Verification items for the finished model (mm, model axes). A direction names the side the tool comes from. Coordinates: 2 decimals unless noted, no trailing zeros. Loops run counter-clockwise (first coordinate to the right, second up) from the corner with the lowest first, then second, coordinate; pieces in that order, holes last. Notation, with made-up numbers: (35, 6) - (46, 6) arc R20 cw to (46, 33) - close; hole circle Ø5 at (20, -15.75). An arc over 180 degrees is marked (long way). Answer as CSV lines item,"result". Start each with the question number.
1. Set-up check for faces 1 (the flat face through (2, 5.562, 0)), 2 (the cylindrical face through (2.539, -3.023, 17.085)): record each of +Z, -Z, +X, -X, +Y, -Y from which the full face is reachable in a straight line by a thin tool's end or side.
2. Cross-section at C-C (x = 3.75). State how many separate pieces and enclosed holes the cut face has, plus the area to 3 significant figures.
3. Gauge pin test, flat ends, axial feed: P1, Ø0.8, axis at x = 3.5, z = 0, coming from the -Y side; P2, Ø12, axis at y = -11.5, z = 14, coming from the +X side; P3, Ø1.5, axis at x = 3, y = -6, coming from the +Z side; P4, Ø1.5, axis at y = 0, z = 7.5, coming from the -X side. Record the tip position at first contact, or that the pin passes through.
4. Material ranges on line 1 (Y direction, x = 2.5, z = 0) (3 decimals); line 2 (Z direction, x = 0.35, y = 2.5); line 3 (Z direction, x = 1.85, y = 9), recorded low to high. Write a range as [from, to].
5. Cross-section at A-A (y = 0). Enter the section's corners in (x, z) (3 decimals), plus the area to 3 significant figures.
6. Release check for a two-part mould opening along Y. For faces 3 (the cylindrical face through (2.539, 8.684, -15.02)), 4 (the flat face through (2.46, 2.79, 4.81)), 5 (the flat face through (2.465, 8.988, 3.874)), 6 (the cylindrical face through (2.54, -4.48, -16.76)) record: pulls with the +Y half, pulls with the -Y half, needs draft (parallel to the pull), parting line crosses it, or undercut.
```python
from build123d import *

# Parameters (mm, degrees)
SKETCH1_R           = 20
SKETCH1_R_2         = 1.705
BOSS_EXTRUDE1_DEPTH = 5
CUT_EXTRUDE1_DEPTH  = 8
CIRPATTERN1_COUNT   = 12
CUT_EXTRUDE2_DEPTH  = 2.5
CIRPATTERN2_COUNT   = 71
CIRPATTERN2_ANGLE   = 350


with BuildPart() as part:
    # Sketch1 → Boss-Extrude1 (new body)
    with BuildSketch(Plane(origin=(0, 0, 0), x_dir=(0, 0, -1), z_dir=(1, 0, 0))):
        Circle(SKETCH1_R)
        Circle(SKETCH1_R_2, mode=Mode.SUBTRACT)
    extrude(amount=BOSS_EXTRUDE1_DEPTH)

    # Sketch2 → Cut-Extrude1 (cut)
    with BuildSketch(Plane(origin=(0, 0, 0), x_dir=(0, 0, -1), z_dir=(1, 0, 0))):
        with BuildLine():
            Line((1.467292325, 13.76439168), (0.800439906, 5.562312437))
            Line((0.800439906, 5.562312437), (-0.800439906, 5.562312437))
            Line((-0.800439906, 5.562312437), (-1.467292325, 13.76439168))
            ThreePointArc((-1.467292325, 13.76439168), (0, 15.231684005), (1.467292325, 13.76439168))
        make_face()
    cut_extrude1 = extrude(amount=CUT_EXTRUDE1_DEPTH, mode=Mode.SUBTRACT)

    # CirPattern1: Cut-Extrude1 ×12 about axis
    cirpattern1_axis = Axis((0, 0, 0), (1, 0, 0))
    for i in range(1, CIRPATTERN1_COUNT):
        add(cut_extrude1.rotate(cirpattern1_axis, i * 360 / CIRPATTERN1_COUNT), mode=Mode.SUBTRACT)

    # Sketch6 → Cut-Extrude2 (cut, symmetric)
    with BuildSketch(Plane.XY):
        with BuildLine():
            Line((0, 16.3), (0, 20))
            Line((0, 20), (5, 20))
            Line((5, 20), (5, 16.3))
            ThreePointArc((5, 16.3), (2.5, 17.350510257), (0, 16.3))
        make_face()
    cut_extrude2 = extrude(amount=CUT_EXTRUDE2_DEPTH, both=True, mode=Mode.SUBTRACT)

    # CirPattern2: Cut-Extrude2 ×71 about axis
    cirpattern2_axis = Axis((5, 0, 0), (-1, 0, 0))
    for i in range(1, CIRPATTERN2_COUNT):
        add(cut_extrude2.rotate(cirpattern2_axis, i * CIRPATTERN2_ANGLE / (CIRPATTERN2_COUNT - 1)), mode=Mode.SUBTRACT)


solid = part.part
```
Values follow:
1,face 1,"+X, -X"
1,face 2,"+Z, -Y"
2,separate pieces,"1"
2,enclosed holes,"13"
2,area,"648 mm²"
3,P1,"stops at y = -17.3"
3,P2,"stops at x = 5"
3,P3,"stops at z = 16.53"
3,P4,"passes through"
4,line 1,"y = [-17.351, -15.232], [-5.562, -1.705], [1.705, 5.562], [15.232, 17.351]"
4,line 2,"z = [-16.43, -6.09], [-4.98, 4.98], [6.09, 16.43]"
4,line 3,"z = [-14.77, -6.64], [-3.88, -1.08], [1.08, 3.88], [6.64, 14.77]"
5,outline,"(0, -16.3) arc R3.5 ccw to (5, -16.3) - (5, -15.232) - (0, -15.232) - close; (0, -5.562) - (5, -5.562) - (5, -1.705) - (0, -1.705) - close; (0, 1.705) - (5, 1.705) - (5, 5.562) - (0, 5.562) - close; (0, 15.232) - (5, 15.232) - (5, 16.3) arc R3.5 ccw to (0, 16.3) - close"
5,area,"56.5 mm²"
6,face 3,"pulls with the +Y half"
6,face 4,"undercut"
6,face 5,"undercut"
6,face 6,"pulls with the -Y half"
